Here's how the part is built. I have some questions about the finished solid (model axes, mm). A direction names the side the tool comes from. Round coordinates to 2 decimals unless told otherwise and drop trailing zeros. Write each loop counter-clockwise with the first axis right and the second up, starting at its lowest first coordinate (ties: lowest second). Pieces come first, ordered by that corner, then holes. Notation, with made-up numbers: (-8, 17.25) - (15, 17.25) arc R20 ccw to (15, 53.25) - close; hole circle Ø2 at (59.5, -26.75). An arc over 180 degrees is marked (long way). One line per question, with ' | ' between items. Start each with the question number.
(1) Will these pins go through, and if not, where does the flat tip stop? pin 1 (4 mm diameter, centred on x = -24, y = 14, fed in from -Z); pin 2 (1.2 mm diameter, centred on x = -34, z = 1, fed in from +Y).
(2) Imagine slicing it at D-D (x = -27). Write out the boundary of the cut face in (y, z).
(3) Imagine slicing it at B-B (x = -4). Write out the boundary of the cut face in (y, z), plus the area to 3 significant figures.
(4) Imagine slicing it at A-A (z = 3.15). Write out the boundary of the cut face in (x, y).
(5) Imagine slicing it at C-C (y = 22). Write out the boundary of the cut face in (x, z), plus the area to 3 significant figures.
(6) Thinking about a two-plate mould opening in X: for faces 1 (the flat face through (-1.5, 25, 1)), 2 (the flat face through (-33, 37, 0)), 3 (the cylindrical face through (-0.764, 46.84, 2.028)), which applies, pulls with the +X half, pulls with the -X half, needs draft (parallel to the pull), parting line crosses it, or undercut?
(7) If I drill on L1, parallel to Y at x = -6.5, z = 3.35; L2, parallel to X at y = 6.5, z = 2.9; L3, parallel to Z at x = -15, y = 3.5, over which ranges is the centre line in solid material (lowest first)?
(8) For faces 4 (the flat face through (-26, 1.5, 1)), 5 (the flat face through (-26, 0, 2)), which set-ups out of +Z, -Z, +X, -X, +Y, -Y let a thin tool reach every point of the face, with its end or its side?
from build123d import *

# Parameters (mm, degrees)
F1_DEPTH = 4
F2_T     = -1.5
F5_DEPTH = 2.5
F6_R     = 1.5
F7_R     = 3
F9_DEPTH = 4.001


with BuildPart() as f1:
    # F0 (on Top) → F1 (new body)
    with BuildSketch(Plane.XY):
        with BuildLine():
            ThreePointArc((-6.5, 0), (-1.9038059223, 1.9038059223), (0, 6.5))
            Line((0, 6.5), (0, 47.4878030638))
            ThreePointArc((0, 47.4878030638), (-35.8449314192, 35.8449314192), (-47.4878030638, 0))
            Line((-47.4878030638, 0), (-13, 0))
            Line((-13, 0), (-6.5, 0))
        make_face()
    extrude(amount=F1_DEPTH)

    # F2
    f2_openings = [f1.faces().sort_by_distance(p)[0] for p in [
        (-21.274509, 21.274509, 4),
        (-21.274509, 21.274509, 0),
    ]]
    offset(amount=F2_T, openings=f2_openings)

    # F4 (on offset) → F5 (join)
    with BuildSketch(Plane.XY.offset(1.5)):
        with BuildLine():
            Line((-46.186269666, 1.5), (-6.5, 1.5))
            ThreePointArc((-6.5, 1.5), (-2.9644660941, 2.9644660941), (-1.5, 6.5))
            Line((-1.5, 6.5), (-1.5, 46.186269666))
            ThreePointArc((-1.5, 46.186269666), (-34.7842712475, 34.7842712475), (-46.186269666, 1.5))
        make_face()
    extrude(amount=F5_DEPTH)

    # F6
    f6_edges = [f1.edges().sort_by_distance(p)[0] for p in [
        (-1.5, 46.18627, 0.75),
        (-46.18627, 1.5, 0.75),
    ]]
    fillet(f6_edges, radius=F6_R)

    # F7
    f7_edges = [f1.edges().sort_by_distance(p)[0] for p in [
        (-47.487803, 0, 2),
        (0, 47.487803, 2),
    ]]
    fillet(f7_edges, radius=F7_R)

    # F8 (on face) → F9 (cut, through all)
    with BuildSketch(Plane(origin=(0, 0, 0), x_dir=(1, 0, 0), z_dir=(0, 0, -1))):
        with BuildLine():
            ThreePointArc((-1.5, -6.5), (-2.9644660941, -2.9644660941), (-6.5, -1.5))
            ThreePointArc((-6.5, -1.5), (-10.0355339059, -10.0355339059), (-1.5, -6.5))
        make_face()
    extrude(amount=-F9_DEPTH, mode=Mode.SUBTRACT)


solid = f1.part
Check sheet entries:
1) pin 1: z = 1.5 | pin 2: y = 38.1
2) outline: (0, 0) - (1.5, 0) - (1.5, 1.5) - (40.85, 1.5) - (40.85, 0) - (42.58, 0) - (42.58, 4) - (0, 4) - close
3) outline: (0.5, 0) - (2.17, 0) - (2.17, 4) - (0.5, 4) - close; (10.83, 1.5) - (46.42, 1.5) - (46.42, 0) - (47.92, 0) - (47.92, 4) - (10.83, 4) - close | area: 102 mm^2
4) outline: (-47.83, 2.73) arc R3 ccw to (-44.84, 0) - (-6.5, 0) arc R6.5 ccw to (0, 6.5) - (0, 44.84) arc R3 ccw to (-2.73, 47.83) arc R41.5 ccw to start; hole circle Ø10 at (-6.5, 6.5)
5) outline: (-45, 0) - (-43.37, 0) - (-43.37, 1.5) - (-1.5, 1.5) - (-1.5, 0) - (0, 0) - (0, 4) - (-45, 4) - close | area: 117 mm^2
6) face 1: undercut | face 2: needs draft | face 3: pulls with the +X half
7) L1: 0 to 1.5, 11.5 to 48 | L2: -48 to -11.5, -1.5 to 0 | L3: 1.5 to 4
8) face 4: -Z | face 5: +Z, -Z, +X, -X, -Y
